Model file for the job. Use its own axes, mm. Face numbers are marked on the shaded views. Coordinates: 2 decimals unless noted, no trailing zeros. Write each loop counter-clockwise with the first axis right and the second up, starting at its lowest first coordinate (ties: lowest second). Pieces come first, ordered by that corner, then holes.
Q1. Pull direction X, two halves, no side cores. Call the marked faces 1, 2 and 3: released by +X, released by -X, zero draft, split by the parting line, or undercut.
Q2. Band-saw the part on D-D, the plane x = 8. Write the cut outline in (y, z), plus the area to 4 significant figures.
Q3. Drill centre lines: probe 1 along X at (y, z) = (2.5, 0); probe 2 along X at (y, z) = (0.75, -22.5); probe 3 along Y at (x, z) = (32, 2.5). Where is each one in solid material? Low to high.
Q4. Band-saw the part on A-A, the plane z = -14. Write the cut outline in (x, y).
Q5. Band-saw the part on B-B, the plane x = -2. Write the cut outline in (y, z).
Q6. Band-saw the part on C-C, the plane y = 4.75. Write the cut outline in (x, z).
Q7. Pin check, flat tips, straight feed: P1, Ø1, axis at y = 2, z = -4.5, coming from the -X side; P2, Ø1, axis at x = 32, y = 1, coming from the +Z side; P3, Ø2, axis at x = -6.5, z = -10.5, coming from the +Y side; P4, Ø4, axis at y = 1, z = -9, coming from the +X side. Stop position of each tip, or through.
Autodesk Inventor part; units mm, degrees
ref_plane "YZ Plane" through (0, 0, 0) normal (1, 0, 0) x (0, 1, 0)
ref_plane "XZ Plane" through (0, 0, 0) normal (0, 1, 0) x (-1, 0, 0)
ref_plane "XY Plane" through (0, 0, 0) normal (0, 0, 1) x (1, 0, 0)
sketch "Sketch5" plane through (0, 0, 0) normal (0, 1, 0) x (-1, 0, 0)
  line L0 (9.4203, 11.6048) -> (-50.5797, 11.6048)
  line L1 (-50.5797, 11.6048) -> (-50.5797, -27.8952)
  line L2 (-50.5797, -27.8952) -> (9.4203, -27.8952)
  line L3 (9.4203, -27.8952) -> (9.4203, 11.6048)
  line L4 (-33.3686, -23.1452) -> (-31.3686, -23.1452)
  line L5 (-31.3686, -23.1452) -> (-31.3686, 6.8548)
  line L6 (-31.3686, 6.8548) -> (-33.3686, 6.8548)
  line L7 (-33.3686, 6.8548) -> (-33.3686, -23.1452)
  line L8 (7.9203, 6.8548) -> (5.9203, 6.8548)
  line L9 (5.9203, 6.8548) -> (5.9203, -23.1452)
  line L10 (5.9203, -23.1452) -> (7.9203, -23.1452)
  line L11 (7.9203, -23.1452) -> (7.9203, 6.8548)
  circle A0 centre (2.9203, -21.3952) radius 1.5
  circle A1 centre (2.9203, 5.1048) radius 1.5
  circle A2 centre (-34.8686, -25.3952) radius 1.5
  circle A3 centre (-34.8686, 9.1048) radius 1.5
  point P0 (0, 0)
  dimension "d9" = 60
  dimension "d10" = 39.5
  dimension "d24" = 2
  dimension "d27" = 4.75
  dimension "d29" = 2
  dimension "d31" = 1.5
  dimension "d32" = 4.75
  dimension "d33" = 4.75
  dimension "d40" = 3
  dimension "d41" = 6.5
  dimension "d42" = 6.5
  dimension "d43" = 3
  dimension "d44" = 6.5
  dimension "d45" = 6.5
  dimension "d46" = 3
  dimension "d47" = 2.5
  dimension "d49" = 3
  dimension "d50" = 2.5
  dimension "d59" = 35
  dimension "d62" = 1.5
  dimension "d66" = 35
extrude "Extrusion8" add sketch "Sketch5" against normal blind 1.5 contours L3 L2 L1 L0 | L7 L6 L5 L4 | L11 L10 L9 L8 | A0 | A1 | A2 | A3
extrude "Extrusion9" add sketch "Sketch5" along normal blind 3.5 contours L7 L6 L5 L4 | L11 L10 L9 L8
extrude "Extrusion10" add sketch "Sketch5" along normal blind 6 contours A0 | A1 | A2 | A3
properties part number "RFID-RC522 Holder 3.2"
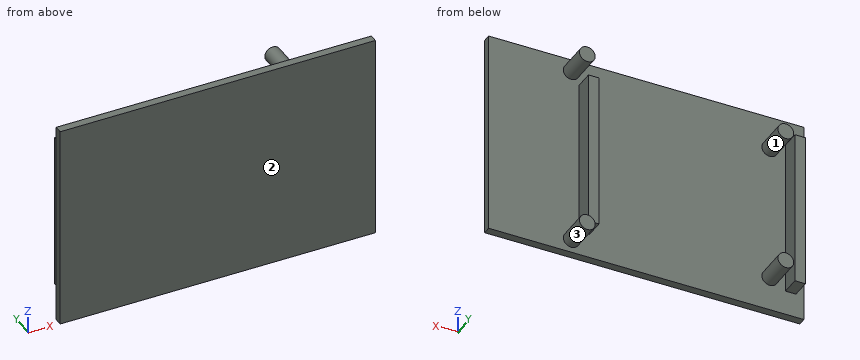
Answer sheet:
1. face 1: undercut
1. face 2: zero draft
1. face 3: split by the parting line
2. outline: (-1.5, -27.9) - (0, -27.9) - (0, 11.6) - (-1.5, 11.6) - close
2. area: 59.25 mm2
3. probe 1: x = -7.92 to -5.92, 31.37 to 33.37
3. probe 2: x = -7.92 to -5.92, -3.93 to -1.91, 31.37 to 33.37
3. probe 3: y = -1.5 to 3.5
4. outline: (-9.42, -1.5) - (50.58, -1.5) - (50.58, 0) - (33.37, 0) - (33.37, 3.5) - (31.37, 3.5) - (31.37, 0) - (-5.92, 0) - (-5.92, 3.5) - (-7.92, 3.5) - (-7.92, 0) - (-9.42, 0) - close
5. outline: (-1.5, -27.9) - (0, -27.9) - (0, -22.58) - (6, -22.58) - (6, -20.21) - (0, -20.21) - (0, 3.92) - (6, 3.92) - (6, 6.29) - (0, 6.29) - (0, 11.6) - (-1.5, 11.6) - close
6. outline: circle Ø3 at (-2.92, -21.4); circle Ø3 at (-2.92, 5.1); circle Ø3 at (34.87, -25.4); circle Ø3 at (34.87, 9.1)
7. P1: stops at x = -7.92
7. P2: stops at z = 6.85
7. P3: stops at y = 3.5
7. P4: stops at x = 50.58
